Could you check a few things on this model? Use its own coordinates, in mm. A direction names the side the tool comes from. Give positions to 0.01 mm unless a question says otherwise; leave off trailing zeros. Loops run counter-clockwise (first coordinate to the right, second up) from the corner with the lowest first, then second, coordinate; pieces in that order, holes last. Notation, with made-up numbers: (-21, 81.5) - (24, 81.5) arc R17 cw to (24, 98.5) - close; hole circle Ø6 at (17.5, 69.5). An arc over 180 degrees is marked (long way). Write each question's results on one line, items separated by ' | '. Start each with the question number.
(1) For pin 1 (18 mm diameter, centred on x = -6, z = 22, fed in from +Y); pin 2 (12 mm diameter, centred on y = 63.5, z = 10.5, fed in from +X); pin 3 (18 mm diameter, centred on x = -3.5, z = -13.5, fed in from -Y), each with a flat end and sliding along its axis, tell me the tip position at first contact or that it passes through.
(2) Suppose I cut it at A-A (x = 62.5). Please give me the cut outline in (y, z).
(3) If we mould it in two halves opening along Y, with no side actions, what happens to faces 4 (the face through (-1, 5, -30)), 5 (the face through (-50, 20, -1)), 6 (the face through (0, 85, -25))? For each: released by +Y, released by -Y, zero draft, split by the parting line, or undercut.
(4) On a 3-axis mill with a long thin cutter (end or side, diameter ignored), from which of +Z, -Z, +X, -X, +Y, -Y can I reach the whole of each face in a straight line? I mean faces 1 (the face through (68, 15, 7.5)), 2 (the face through (0, 25, 6)), 3 (the face through (-67, 15, -7.5)). Say none if no direction works.
(5) Suppose I cut it at B-B (z = -26). Please give me the cut outline in (x, y), and give its area (3 significant figures).
(6) Suppose I cut it at C-C (y = 53.5). Please give me the cut outline in (x, z), and give its area (3 significant figures).
(7) I need wall thicknesses on line 1 (X direction, y = 78.5, z = -36); line 2 (Y direction, x = 28, z = -38.5); line 3 (Y direction, x = 0, z = -43). Which ranges of each line are inside material? Lowest first, please.
(8) Suppose I cut it at D-D (x = 0). Please give me the cut outline in (y, z), and give its area (3 significant figures).
from build123d import *

# Parameters (mm, degrees)
SKETCH1_W           = 150
SKETCH1_H           = 100
BOSS_EXTRUDE1_DEPTH = 20
SKETCH2_W           = 60
SKETCH2_H           = 10
CUT_EXTRUDE1_DEPTH  = 151
CUT_EXTRUDE2_DEPTH  = 20
BOSS_EXTRUDE3_DEPTH = 40
SKETCH10_W          = 60
SKETCH10_H          = 60
CUT_EXTRUDE3_DEPTH  = 90
SKETCH11_R          = 15
CUT_EXTRUDE4_DEPTH  = 90


with BuildPart() as part:
    # Sketch1 → Boss-Extrude1 (new body)
    with BuildSketch(Plane(origin=(0, 0, 0), x_dir=(1, 0, 0), z_dir=(0, 1, 0))):
        Rectangle(SKETCH1_W, SKETCH1_H)
    extrude(amount=BOSS_EXTRUDE1_DEPTH)

    # Sketch2 → Cut-Extrude1 (cut, through all)
    with BuildSketch(Plane.ZY.offset(75)):
        with Locations((0, 5)):
            Rectangle(SKETCH2_W, SKETCH2_H)
    extrude(amount=-CUT_EXTRUDE1_DEPTH, mode=Mode.SUBTRACT)

    # Sketch3 → Cut-Extrude2 (cut)
    with BuildSketch(Plane(origin=(0, 20, 0), x_dir=(1, 0, 0), z_dir=(0, 1, 0))):
        with BuildLine():
            Line((-75, 7.5), (-75, -7.5))
            Line((-75, -7.5), (-60, -7.5))
            ThreePointArc((-60, -7.5), (-52.5, 0), (-60, 7.5))
            Line((-60, 7.5), (-75, 7.5))
        make_face()
        with BuildLine():
            Line((75, 7.5), (75, -7.5))
            Line((75, -7.5), (60, -7.5))
            ThreePointArc((60, -7.5), (52.5, 0), (60, 7.5))
            Line((60, 7.5), (75, 7.5))
        make_face()
    extrude(amount=-CUT_EXTRUDE2_DEPTH, mode=Mode.SUBTRACT)

    # Sketch8 → Boss-Extrude3 (add, symmetric)
    with BuildSketch(Plane(origin=(0, 0, 0), x_dir=(0, 0, -1), z_dir=(1, 0, 0))):
        Polygon((50, 20), (50, 100), (30, 100), (-50, 40), (-50, 20), align=None)
    extrude(amount=BOSS_EXTRUDE3_DEPTH, both=True)

    # Sketch10 → Cut-Extrude3 (cut)
    with BuildSketch(Plane.XY.offset(50)):
        with Locations((0, 55)):
            Rectangle(SKETCH10_W, SKETCH10_H)
    extrude(amount=-CUT_EXTRUDE3_DEPTH, mode=Mode.SUBTRACT)

    # Sketch11 → Cut-Extrude4 (cut)
    with BuildSketch(Plane(origin=(0, 0, -50), x_dir=(-1, 0, 0), z_dir=(0, 0, -1))):
        with Locations((0, 60)):
            Circle(SKETCH11_R)
    extrude(amount=-CUT_EXTRUDE4_DEPTH, mode=Mode.SUBTRACT)


solid = part.part
Output values:
1) pin 1: y = 25 | pin 2: x = 40 | pin 3: y = 10
2) outline: (0, -50) - (20, -50) - (20, -7.5) - (10, -7.5) - (10, -30) - (0, -30) - close; (0, 30) - (10, 30) - (10, 7.5) - (20, 7.5) - (20, 50) - (0, 50) - close
3) face 4: zero draft | face 5: released by +Y | face 6: undercut
4) face 1: +X, +Y, -Y | face 2: +Z | face 3: -X, +Y, -Y
5) outline: (-75, 10) - (75, 10) - (75, 20) - (40, 20) - (40, 97) - (-40, 97) - (-40, 20) - (-75, 20) - close; hole (-30, 25) - (30, 25) - (30, 85) - (-30, 85) - close | area: 4,060 mm2
6) outline: (-40, -50) - (-13.52, -50) - (-13.52, -40) - (-30, -40) - (-30, 32) - (-40, 32) - close; (13.52, -50) - (40, -50) - (40, 32) - (30, 32) - (30, -40) - (13.52, -40) - close | area: 1,970 mm2
7) line 1: -40 to -30, 30 to 40 | line 2: 0 to 25, 85 to 100 | line 3: 0 to 45, 75 to 100
8) outline: (0, -50) - (45, -50) - (45, -40) - (25, -40) - (25, 50) - (0, 50) - (0, 30) - (10, 30) - (10, -30) - (0, -30) - close; (75, -50) - (100, -50) - (100, -30) - (85, -10) - (85, -40) - (75, -40) - close | area: 2,650 mm2
